from build123d import *

# Parameters (mm, degrees)
BOSS_EXTRUDE1_DEPTH = 4.5
FILLET1_R           = 10
BOSS_EXTRUDE2_DEPTH = 4.5
FILLET2_R           = 30
SKETCH3_R           = 2.5
CUT_EXTRUDE1_DEPTH  = 5


with BuildPart() as part:
    # Sketch1 → Boss-Extrude1 (new body)
    with BuildSketch(Plane.XY):
        Polygon((10, -15), (10, 0), (10, 15), (15, 15), (15, 35), (10, 35), (10, 50), (-15, 50), (-15, -50), (10, -50), (10, -35), (15, -35), (15, -15), align=None)
    extrude(amount=BOSS_EXTRUDE1_DEPTH)

    # Fillet1
    fillet1_edges = [part.edges().sort_by_distance(p)[0] for p in [
        (-15, -50, 2.25),
        (-15, 50, 2.25),
    ]]
    fillet(fillet1_edges, radius=FILLET1_R)

    # Sketch2 → Boss-Extrude2 (add)
    with BuildSketch(Plane.XY.offset(4.5)):
        with BuildLine():
            Line((-40, 0), (-13.630305493, 45.051517306))
            ThreePointArc((-13.630305493, 45.051517306), (-14.651503897, 42.616958642), (-15, 40))
            Line((-15, 40), (-15, -40))
            ThreePointArc((-15, -40), (-12.071067812, -47.071067812), (-5, -50))
            Line((-5, -50), (-40, -50))
            Line((-40, -50), (-40, 0))
        make_face()
    extrude(amount=-BOSS_EXTRUDE2_DEPTH)

    # Fillet2
    fillet2_edges = [part.edges().sort_by_distance(p)[0] for p in [
        (-40, -50, 2.25),
        (-40, 0, 2.25),
    ]]
    fillet(fillet2_edges, radius=FILLET2_R)

    # Sketch3 → Cut-Extrude1 (cut)
    with BuildSketch(Plane.XY.offset(4.5)):
        with Locations((-20, -35)):
            Circle(SKETCH3_R)
    extrude(amount=-CUT_EXTRUDE1_DEPTH, mode=Mode.SUBTRACT)


solid = part.part
Verification items for the finished model (mm, model axes). A direction names the side the tool comes from. Coordinates: 2 decimals unless noted, no trailing zeros. Order: outer loops, then holes, each group sorted by start corner. A loop starts at its lowest first (then second) coordinate and runs counter-clockwise, first axis right, second up. Notation, with made-up numbers: M -2,-26 L 33,-26 A12 ccw 33,-11 Z; hole C -28.5,2.25 d8. An arc over 180 degrees is marked long. Return JSON: item names as keys, results as strings.
1) Cross-section at B-B, the plane z = 2.6. Record the boundary of the cut face in (x, y).
Answer list:
{"outline": "M -40,-20 A30 ccw -10,-50 L 10,-50 L 10,-35 L 15,-35 L 15,-15 L 10,-15 L 10,15 L 15,15 L 15,35 L 10,35 L 10,50 L -5,50 A10 ccw -13.63,45.05 L -35.89,7.02 A30 ccw -40,-8.13 Z; hole C -20,-35 d5"}
2) Release check for a two-part mould opening along Y. For faces 1 (the flat face through (13, -15, 2)), 2 (the flat face through (-12, 1, 4.5)), 3 (the flat face through (10, 0, 2)), 4 (the cylindrical face through (-9.91, 48.71, 2.28)) record: +Y half, -Y half, draft (parallel to the pull), parting line (faces both ways), or undercut.
Answer list:
{"face 1": "undercut", "face 2": "draft", "face 3": "undercut", "face 4": "+Y half"}
3) Cross-section at C-C, the plane y = 4. Record the boundary of the cut face in (x, z), and give its area (3 significant figures).
Answer list:
{"outline": "M -37.44,0 L 10,0 L 10,4.5 L -37.44,4.5 Z", "area": "213 mm2"}
4) Cross-section at D-D, the plane y = 42.5. Record the boundary of the cut face in (x, z).
Answer list:
{"outline": "M -15.12,0 L 10,0 L 10,4.5 L -15.12,4.5 Z"}
5) Cross-section at A-A, the plane x = -20. Record the boundary of the cut face in (y, z), and give its area (3 significant figures).
Answer list:
{"outline": "M -48.28,0 L -37.5,0 L -37.5,4.5 L -48.28,4.5 Z; M -32.5,0 L 34.17,0 L 34.17,4.5 L -32.5,4.5 Z", "area": "349 mm2"}
6) Gauge pin test, flat ends, axial feed: pin 1 (2 mm diameter, centred on y = -2.5, z = 1, fed in from +X); pin 2 (2 mm diameter, centred on x = 13.5, z = 2, fed in from -Y); pin 3 (2 mm diameter, centred on x = 13, z = 2.5, fed in from +Y). Record the tip position at first contact, or that the pin passes through.
Answer list:
{"pin 1": "x = 10", "pin 2": "y = -35", "pin 3": "y = 35"}
7) Access from +Z, -Z, +X, -X, +Y, -Y to the whole of each face (thin tool, end or side, straight path). Record for faces 5 (the flat face through (13, 35, 2)), 6 (the cylindrical face through (-38.925, -0.176, 2.218)), 7 (the flat face through (12, -35, 2)), 8 (the cylindrical face through (-30.979, -41.445, 2.218)), 9 (the flat face through (12, 15, 2)).
Answer list:
{"face 5": "+Z, -Z, +X, +Y", "face 6": "+Z, -Z, -X, +Y", "face 7": "+Z, -Z, +X, -Y", "face 8": "+Z, -Z, -X, -Y", "face 9": "+Z, -Z, +X"}
8) Thickness scan on L1, parallel to Y at x = 10.5, z = 3.85; L2, parallel to Y at x = -20, z = 2.5; L3, parallel to X at y = -43.5, z = 2.35. Record the ranges inside material, lowest first. Write a range as [from, to].
Answer list:
{"L1": "[-35, -15], [15, 35]", "L2": "[-48.28, -37.5], [-32.5, 34.17]", "L3": "[-28.65, 10]"}
